For this review, take the finished solid that the model builds, in its own axes (mm). Face numbers are marked on the shaded views. A direction names the side the tool comes from. Round coordinates to 2 decimals unless told otherwise and drop trailing zeros. Order: outer loops, then holes, each group sorted by start corner. A loop starts at its lowest first (then second) coordinate and runs counter-clockwise, first axis right, second up. Notation, with made-up numbers: (51, 72.5) -> (69, 72.5) arc R21 ccw to (69, 89.5) -> close; hole circle Ø10 at (24, 74). An arc over 180 degrees is marked (long way). Use a Markdown table: item, result. Add a question column.
1) Machinability: for the marked faces 1 and 2, which of the approach directions +Z, -Z, +X, -X, +Y, -Y give a long, thin tool a straight path to every point of the face, cutting with its end or side? Answer none if there is none.
2) Consider section C-C (x = 21). State the section outline as (y, z) points, plus the area to 3 significant figures.
3) Wall thickness on line 1 along X through (y, z) = (1.4, 4); line 2 along Z through (x, y) = (16.5, 4.55); line 3 along Z through (x, y) = (20.75, 4.35): over which ranges is each line inside the solid? List them lowest first. Write a range as [from, to].
4) Consider section D-D (y = 3.85). State the section outline as (x, z) points.
5) Consider section B-B (z = -21). State the section outline as (x, y) points, plus the area to 3 significant figures.
6) Draft analysis for pull direction Z (two halves, no side actions). For the marked faces 3, 4 and 5, state which applies: pulls with the +Z half, pulls with the -Z half, needs draft (parallel to the pull), parting line crosses it, or undercut.
7) Consider section A-A (y = 0.45). State the section outline as (x, z) points.
8) Clearance check with a flat-ended pin moving along its axis: P1, Ø5, axis at x = 7, z = -4.5, coming from the +Y side. State where the tip first meets the part, or that it passes through.
```python
from build123d import *

# Parameters (mm, degrees)
SKETCH1_W           = 22
SKETCH1_H           = 17
BOSS_EXTRUDE1_DEPTH = 2
SKETCH1_3_W         = 28
SKETCH1_3_H         = 33
SKETCH1_3_R         = 1.75
SKETCH1_3_W_2       = 22
SKETCH1_3_H_2       = 17
BOSS_EXTRUDE2_DEPTH = 6


with BuildPart() as part:
    # Sketch1 → Boss-Extrude1 (new body)
    with BuildSketch(Plane(origin=(0, 0, 0), x_dir=(1, 0, 0), z_dir=(0, 1, 0))):
        with Locations((11, 8.5)):
            Rectangle(SKETCH1_W, SKETCH1_H)
    extrude(amount=BOSS_EXTRUDE1_DEPTH)

    # Sketch1_3 → Boss-Extrude2 (add)
    with BuildSketch(Plane(origin=(0, 0, 0), x_dir=(1, 0, 0), z_dir=(0, 1, 0))):
        with Locations((11, 8.5)):
            Rectangle(SKETCH1_3_W, SKETCH1_3_H)
        with Locations(Location((21, -4, 0), (0, 0, 90))):
            Circle(SKETCH1_3_R, mode=Mode.SUBTRACT)
        with Locations(Location((1, -4, 0), (0, 0, 270))):
            Circle(SKETCH1_3_R, mode=Mode.SUBTRACT)
        with Locations(Location((21, 21, 0), (0, 0, 270))):
            Circle(SKETCH1_3_R, mode=Mode.SUBTRACT)
        with Locations(Location((1, 21, 0), (0, 0, 90))):
            Circle(SKETCH1_3_R, mode=Mode.SUBTRACT)
        with Locations((11, 8.5)):
            Rectangle(SKETCH1_3_W_2, SKETCH1_3_H_2, mode=Mode.SUBTRACT)
    extrude(amount=BOSS_EXTRUDE2_DEPTH)


solid = part.part
```
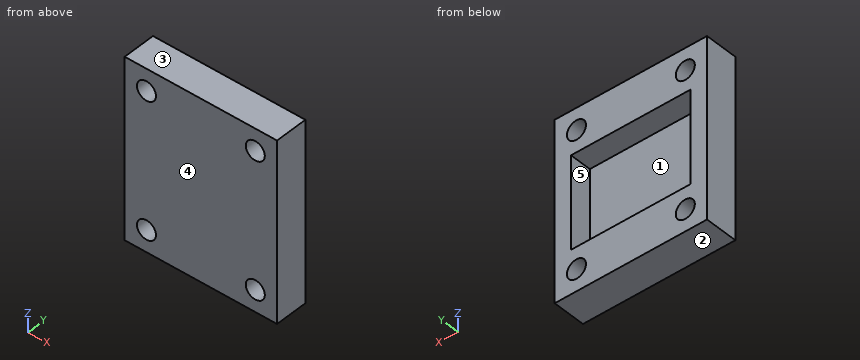
Results list:
| question | item | result |
|---|---|---|
| 1 | face 1 | +Y |
| 1 | face 2 | -Z, +X, -X, +Y, -Y |
| 2 | outline | (0, -25) -> (6, -25) -> (6, -22.75) -> (0, -22.75) -> close; (0, -19.25) -> (6, -19.25) -> (6, -17) -> (2, -17) -> (2, 0) -> (6, 0) -> (6, 2.25) -> (0, 2.25) -> close; (0, 5.75) -> (6, 5.75) -> (6, 8) -> (0, 8) -> close |
| 2 | area | 88.0 mm2 |
| 3 | line 1 | [-3, -0.75], [2.75, 19.25], [22.75, 25] |
| 3 | line 2 | [-25, -17], [0, 8] |
| 3 | line 3 | [-25, -22.73], [-19.27, -17], [0, 2.27], [5.73, 8] |
| 4 | outline | (-3, -25) -> (25, -25) -> (25, 8) -> (-3, 8) -> close; hole circle Ø3.5 at (1, -21); hole circle Ø3.5 at (1, 4); hole (0, -17) -> (22, -17) -> (22, 0) -> (0, 0) -> close; hole circle Ø3.5 at (21, -21); hole circle Ø3.5 at (21, 4) |
| 5 | outline | (-3, 0) -> (-0.75, 0) -> (-0.75, 6) -> (-3, 6) -> close; (2.75, 0) -> (19.25, 0) -> (19.25, 6) -> (2.75, 6) -> close; (22.75, 0) -> (25, 0) -> (25, 6) -> (22.75, 6) -> close |
| 5 | area | 126 mm2 |
| 6 | face 3 | pulls with the +Z half |
| 6 | face 4 | needs draft |
| 6 | face 5 | undercut |
| 7 | outline | (-3, -25) -> (25, -25) -> (25, 8) -> (-3, 8) -> close; hole circle Ø3.5 at (1, -21); hole circle Ø3.5 at (1, 4); hole circle Ø3.5 at (21, -21); hole circle Ø3.5 at (21, 4) |
| 8 | P1 | y = 2 |
